from build123d import *

# Parameters (mm, degrees)
F1_DEPTH = 100
F2_R     = 5


with BuildPart() as f1:
    # F0 (on Front) → F1 (new body)
    with BuildSketch(Plane.XZ):
        Polygon((0, 100), (0, 0), (100, 0), (100, 25), (75, 25), (75, 50), (50, 50), (50, 75), (25, 75), (25, 100), align=None)
    extrude(amount=F1_DEPTH)

    # F2
    f2_edges = [f1.edges().sort_by_distance(p)[0] for p in [
        (25, -50, 100),
        (25, -50, 75),
        (50, -50, 75),
        (50, -50, 50),
        (75, -50, 50),
        (75, -50, 25),
        (100, -50, 25),
        (100, -100, 12.5),
        (100, -50, 0),
        (100, 0, 12.5),
        (87.5, -100, 25),
        (75, -100, 37.5),
        (62.5, 0, 50),
        (62.5, -100, 50),
        (0, -100, 50),
        (50, -100, 0),
        (50, -100, 62.5),
        (37.5, -100, 75),
        (25, -100, 87.5),
        (12.5, -100, 100),
        (0, 0, 50),
        (50, 0, 0),
        (87.5, 0, 25),
        (75, 0, 37.5),
        (50, 0, 62.5),
        (37.5, 0, 75),
        (25, 0, 87.5),
        (12.5, 0, 100),
        (0, -50, 100),
        (0, -50, 0),
    ]]
    fillet(f2_edges, radius=F2_R)


solid = f1.part
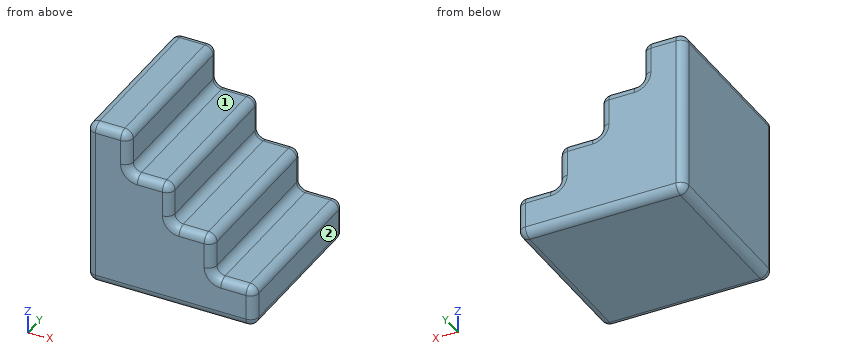
Input: part model. Units: mm. Frame: model coordinates. Face numbers are marked on the shaded views. A direction names the side the tool comes from. Coordinates: 2 decimals unless noted, no trailing zeros. Order: outer loops, then holes, each group sorted by start corner. A loop starts at its lowest first (then second) coordinate and runs counter-clockwise, first axis right, second up. Notation, with made-up numbers: M 87.5,56.25 L 137.5,56.25 A11 cw 137.5,73.25 Z; hole C 66.25,-12 d8. An arc over 180 degrees is marked long. Write item = value, one per line. Start each with the question number.
(1) Section A-A on y = -48. Output: boundary loops of the cut face in (x, z).
(2) First-contact query: P1, Ø7.5, axis at x = 64.5, y = -67, coming from the +Z side; P2, Ø4.5, axis at x = 37, y = -57, coming from the +Z side; P3, Ø12, axis at x = 88.5, y = -31.5, coming from the +Z side. Flat tips, straight axial feed; report the tip coordinate or a pass-through.
(3) Section C-C on z = 68.5. Output: boundary loops of the cut face in (x, y).
(4) Line query: line 1 along X through (y, z) = (-39, 37); line 2 along Z through (x, y) = (66.5, -58.5); line 3 along Z through (x, y) = (4.5, -89.5). Output: solid intervals per line, ascending. Write a range as [from, to].
(5) Reachability of the marked faces 1 and 2 from +Z, -Z, +X, -X, +Y, -Y: full face, straight path, thin tool, end or side. Return the list, or none.
(6) Section B-B on z = 86. Output: boundary loops of the cut face in (x, y), and give its area (3 significant figures).
Result set:
q1.outline = M 0,5 A5 ccw 5,0 L 95,0 A5 ccw 100,5 L 100,20 A5 ccw 95,25 L 80,25 A5 cw 75,30 L 75,45 A5 ccw 70,50 L 55,50 A5 cw 50,55 L 50,70 A5 ccw 45,75 L 30,75 A5 cw 25,80 L 25,95 A5 ccw 20,100 L 5,100 A5 ccw 0,95 Z
q2.P1 = 50
q2.P2 = 75
q2.P3 = 25
q3.outline = M 0,-95 A5 ccw 5,-100 L 45,-100 A5 ccw 50,-95 L 50,-5 A5 ccw 45,0 L 5,0 A5 ccw 0,-5 Z
q4.line_1 = [0, 75]
q4.line_2 = [0, 50]
q4.line_3 = [0.03, 99.97]
q5.face_1 = +Z, +X, +Y, -Y
q5.face_2 = +Z, -Z, +X, +Y, -Y
q6.outline = M 0,-95 A5 ccw 5,-100 L 20,-100 A5 ccw 25,-95 L 25,-5 A5 ccw 20,0 L 5,0 A5 ccw 0,-5 Z
q6.area = 2,480 mm²
